Check sheet for the modelled part. Datum: model origin and axes. Units: mm. A direction names the side the tool comes from. Give positions to 0.01 mm unless a question says otherwise; leave off trailing zeros. Order: outer loops, then holes, each group sorted by start corner. A loop starts at its lowest first (then second) coordinate and runs counter-clockwise, first axis right, second up. Notation, with made-up numbers: (0, 47) -> (6, 47) arc R33 ccw to (6, 82) -> close; hole circle Ø4 at (36.25, -30.75). An arc over 180 degrees is marked (long way). Write each question's results on one line, items separated by ' | '.
from build123d import *

# Parameters (mm, degrees)
F0_W        = 30
F0_H        = 48.5
F0_W_2      = 26
F0_H_2      = 44.5
F1_DEPTH    = 50
F2_W        = 30
F2_H        = 48.5
F3_DEPTH    = 3
F5_DEPTH    = 30
F6_W        = 4
F6_H        = 14
F7_DEPTH    = 20
F8_R        = 0.5
F9_T1_DEPTH = 14
F9_T3_DEPTH = 19


# Not quite as in the source:
# - a fillet or chamfer that OpenCascade refuses, or shapes differently, is made with other operations: its cross-section is extruded or revolved along the edge and cut away or added


with BuildPart() as f1:
    # F0 (on Top) → F1 (new body)
    with BuildSketch(Plane.XY):
        with Locations((13, -22.25)):
            Rectangle(F0_W, F0_H)
        with Locations((13, -22.25)):
            Rectangle(F0_W_2, F0_H_2, mode=Mode.SUBTRACT)
    extrude(amount=F1_DEPTH)

    # F2 (on face) → F3 (join)
    with BuildSketch(Plane(origin=(0, 0, 0), x_dir=(1, 0, 0), z_dir=(0, 0, -1))):
        with Locations((13, 22.25)):
            Rectangle(F2_W, F2_H)
    extrude(amount=F3_DEPTH)

    # F4 (on face) → F5 (cut)
    with BuildSketch(Plane(origin=(-2, 0, 0), x_dir=(0, -1, 0), z_dir=(-1, 0, 0))):
        Polygon((-2, 37), (-2, -3), (28, -3), align=None)
    extrude(amount=-F5_DEPTH, mode=Mode.SUBTRACT)

    # F6 (on face) → F7 (join)
    with BuildSketch(Plane.XY):
        with Locations((15, -32.75)):
            Rectangle(F6_W, F6_H)
        with Locations((11, -32.75)):
            Rectangle(F6_W, F6_H)
    extrude(amount=F7_DEPTH)

    # F8
    f8_edges = [f1.edges().sort_by_distance(p)[0] for p in [
        (0, -35.125, 0),
        (26, -35.125, 0),
        (0, 0, 42.166667),
        (0, -44.5, 25),
        (26, -44.5, 25),
        (26, 0, 42.166667),
    ]]
    fillet(f8_edges, radius=F8_R)

    # F9: fillet of radius 2 on 4 edges, made by hand

    # F9_s2 → F9_t1 (join)
    with BuildSketch(Plane.XZ.offset(25.75)):
        with BuildLine():
            ThreePointArc((19, 0), (17.5857864376, 0.5857864376), (17, 2))
            Line((17, 2), (17, 0))
            Line((17, 0), (19, 0))
        make_face()
        with BuildLine():
            ThreePointArc((7, 0), (8.4142135624, 0.5857864376), (9, 2))
            Line((9, 2), (9, 0))
            Line((9, 0), (7, 0))
        make_face()
    extrude(amount=F9_T1_DEPTH)

    # F9_s4 → F9_t3 (cut)
    with BuildSketch(Plane.XZ.offset(20.75)):
        with BuildLine():
            ThreePointArc((17, 18), (16.4142135624, 19.4142135624), (15, 20))
            Line((15, 20), (17, 20))
            Line((17, 20), (17, 18))
        make_face()
        with BuildLine():
            ThreePointArc((11, 20), (9.5857864376, 19.4142135624), (9, 18))
            Line((9, 18), (9, 20))
            Line((9, 20), (11, 20))
        make_face()
    extrude(amount=F9_T3_DEPTH, mode=Mode.SUBTRACT)


solid = f1.part
1. Section check C-C on z = 44. Record the cut outline in (x, y), then the cut area to 3 significant figures.
Verdict:
outline: (-2, -46.5) -> (28, -46.5) -> (28, 2) -> (-2, 2) -> close; hole (0, -44) arc R0.5 ccw to (0.5, -44.5) -> (25.5, -44.5) arc R0.5 ccw to (26, -44) -> (26, -0.5) arc R0.5 ccw to (25.5, 0) -> (0.5, 0) arc R0.5 ccw to (0, -0.5) -> close | area: 298 mm^2
2. Section check A-A on z = 7. Record the cut outline in (x, y), then the cut area to 3 significant figures.
Verdict:
outline: (-2, -46.5) -> (28, -46.5) -> (28, -20.5) -> (26, -20.5) -> (26, -44) arc R0.5 cw to (25.5, -44.5) -> (0.5, -44.5) arc R0.5 cw to (0, -44) -> (0, -20.5) -> (-2, -20.5) -> close; (9, -39.75) -> (17, -39.75) -> (17, -25.75) -> (9, -25.75) -> close | area: 268 mm^2
3. Mould release check, pull along Y, two halves, no side actions. Record for faces 4 (the flat face through (-2, -27, 30)), 5 (the flat face through (13, -46.5, 24)), 6 (the flat face through (0, -27, 30)), 7 (the flat face through (13, 2, 44)): +Y half, -Y half, draft (parallel to the pull), parting line (faces both ways), or undercut.
Verdict:
face 4: draft | face 5: -Y half | face 6: undercut | face 7: +Y half
4. Gauge pin test, flat ends, axial feed: pin 1 Ø13 at (x, z) = (15.5, 10) entering from +Y; pin 2 Ø4 at (x, y) = (2.5, -21.5) entering from +Z; pin 3 Ø9.5 at (x, y) = (14.5, -30.5) entering from +Z; pin 4 Ø8 at (x, z) = (21.5, 26) entering from +Y. Record the tip position at first contact, or that the pin passes through.
Verdict:
pin 1: stops at y = -25.75 | pin 2: passes through | pin 3: stops at z = 20 | pin 4: stops at y = -44.5
5. Section check D-D on y = -9. Record the cut outline in (x, z).
Verdict:
outline: (-2, 22.33) -> (0, 22.33) -> (0, 50) -> (-2, 50) -> close; (26, 22.33) -> (28, 22.33) -> (28, 50) -> (26, 50) -> close
6. Section check B-B on x = 6. Record the cut outline in (y, z).
Verdict:
outline: (-46.5, -3) -> (-28, -3) -> (-25.75, 0) -> (-44.5, 0) -> (-44.5, 50) -> (-46.5, 50) -> close; (0, 34.33) -> (2, 37) -> (2, 50) -> (0, 50) -> close
7. Material ranges on probe 1 along X at (y, z) = (-26, 11); probe 2 along X at (y, z) = (-29.5, 45); probe 3 along Y at (x, z) = (23.25, 35), recorded low to high. Write a range as from..to.
Verdict:
probe 1: x = -2..0, 9..17, 26..28 | probe 2: x = -2..0, 26..28 | probe 3: y = -46.5..-44.5, 0..0.5
8. Access from +Z, -Z, +X, -X, +Y, -Y to the whole of each face (thin tool, end or side, straight path). Record for faces 1 (the flat face through (13, -25.75, 10)), 2 (the flat face through (13, -44.5, 25)), 3 (the cylindrical face through (16.43, -32.65, 19.4)).
Verdict:
face 1: +Z, -Z, +Y | face 2: +Z | face 3: +Z, +Y
